Verification items for this drawing (mm, ordinates from the low corner). A direction names the side the tool comes from. Round coordinates to 2 decimals unless told otherwise and drop trailing zeros. Order: outer loops, then holes, each group sorted by start corner. A loop starts at its lowest first (then second) coordinate and runs counter-clockwise, first axis right, second up. Notation, with made-up numbers: (6, 41.5) -> (11, 41.5) arc R15 ccw to (11, 61.5) -> close; hole circle Ø11 at (87, 71). An arc over 180 degrees is marked (long way). Answer in a Markdown table with one row per item. Add a question column.
1. Sectioned sample at B-B, the plane x = 10. Record the boundary of the cut face in (y, z), then the cut area to 3 significant figures.
2. Sectioned sample at A-A, the plane x = 5.75. Record the boundary of the cut face in (y, z), then the cut area to 3 significant figures.
3. Depth check by flat-ended pin: P1, Ø3, axis at y = 1, z = 6, coming from the +X side; P2, Ø4, axis at x = 8.5, z = 8.5, coming from the -Y side; P3, Ø0.8, axis at x = 18.5, y = 0.5, coming from the +Z side; P4, Ø1.2, axis at x = 10, y = 2.5, coming from the +Z side. Enter the tip coordinate at first touch or a pass-through.
4. Sectioned sample at C-C, the plane z = 6.5. Record the boundary of the cut face in (x, y), then the cut area to 3 significant figures.
5. Draft check along Z on the marked faces 1, 2, 3 and 4. Enter one of: +Z half, -Z half, draft (parallel to the pull), parting line (faces both ways), or undercut.
6. Material ranges on L1, parallel to Y at x = 11.75, z = 11.25; L2, parallel to X at y = 11, z = 6.75; L3, parallel to Z at x = 10, y = 2, recorded low to high. Write a range as from..to.
7. Sectioned sample at D-D, the plane y = 2.75. Record the boundary of the cut face in (x, z), then the cut area to 3 significant figures.
8. Access from +Z, -Z, +X, -X, +Y, -Y to the whole of each face (thin tool, end or side, straight path). Record for the marked faces 5, 6, 7 and 8.
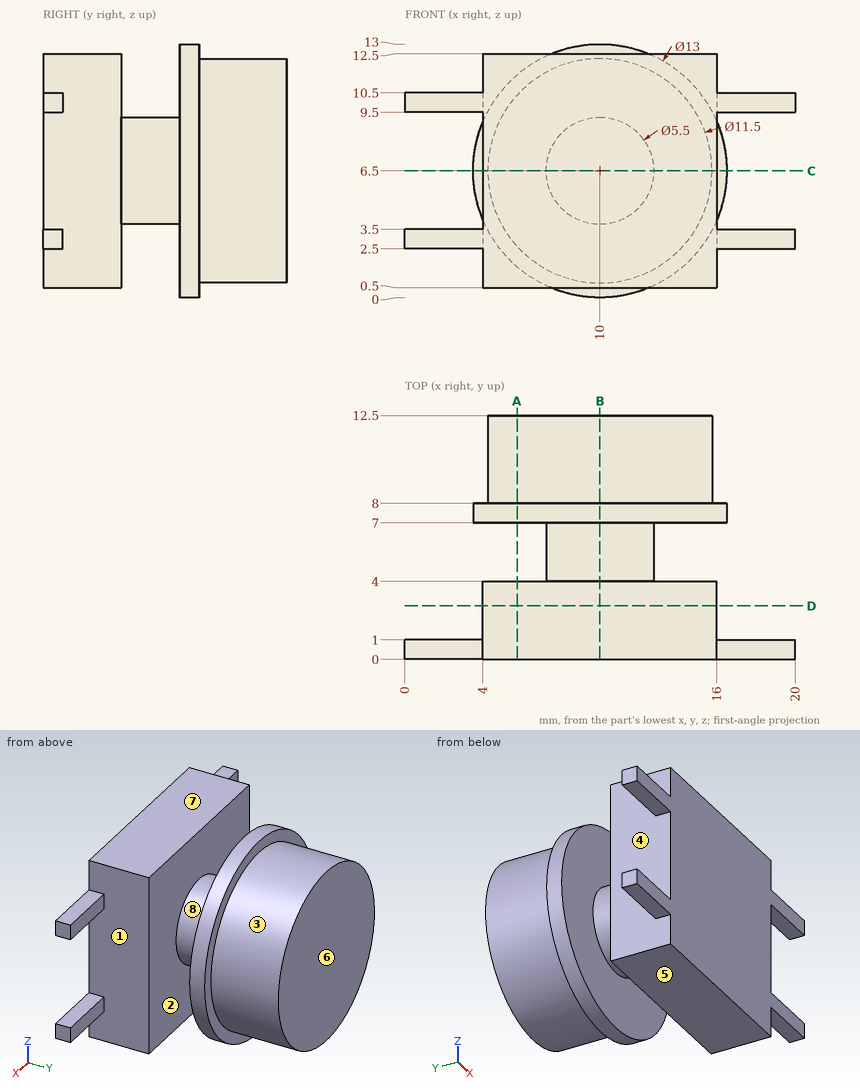
Answer key:
| question | item | result |
|---|---|---|
| 1 | outline | (0, 0.5) -> (4, 0.5) -> (4, 3.75) -> (7, 3.75) -> (7, 0) -> (8, 0) -> (8, 0.75) -> (12.5, 0.75) -> (12.5, 12.25) -> (8, 12.25) -> (8, 13) -> (7, 13) -> (7, 9.25) -> (4, 9.25) -> (4, 12.5) -> (0, 12.5) -> close |
| 1 | area | 129 mm² |
| 2 | outline | (0, 0.5) -> (4, 0.5) -> (4, 12.5) -> (0, 12.5) -> close; (7, 1.58) -> (8, 1.58) -> (8, 2.63) -> (12.5, 2.63) -> (12.5, 10.37) -> (8, 10.37) -> (8, 11.42) -> (7, 11.42) -> close |
| 2 | area | 92.7 mm² |
| 3 | P1 | stops at x = 16 |
| 3 | P2 | stops at y = 0 |
| 3 | P3 | stops at z = 10.5 |
| 3 | P4 | stops at z = 12.5 |
| 4 | outline | (3.5, 7) -> (7.25, 7) -> (7.25, 4) -> (4, 4) -> (4, 0) -> (16, 0) -> (16, 4) -> (12.75, 4) -> (12.75, 7) -> (16.5, 7) -> (16.5, 8) -> (15.75, 8) -> (15.75, 12.5) -> (4.25, 12.5) -> (4.25, 8) -> (3.5, 8) -> close |
| 4 | area | 129 mm² |
| 5 | face 1 | undercut |
| 5 | face 2 | draft |
| 5 | face 3 | parting line |
| 5 | face 4 | undercut |
| 6 | L1 | y = 0..4, 7..12.5 |
| 6 | L2 | x = 4.26..15.74 |
| 6 | L3 | z = 0.5..12.5 |
| 7 | outline | (4, 0.5) -> (16, 0.5) -> (16, 12.5) -> (4, 12.5) -> close |
| 7 | area | 144 mm² |
| 8 | face 5 | -Z, +X, -X, -Y |
| 8 | face 6 | +Z, -Z, +X, -X, +Y |
| 8 | face 7 | +Z, +X, -X, -Y |
| 8 | face 8 | none |
